Autodesk Fusion 360 part; units mm, degrees
sketch "Sketch1" plane through (0, 0, 0) normal (0, 1, 0) x (1, 0, 0)
  circle A0 centre (0, 0) radius 71.65
  circle A1 centre (0, 0) radius 83.65
  circle A2 centre (0, 0) radius 86.15 construction
  line L0 (0, 0) -> (10, 0) construction
  line L1 (-106.5, 0) -> (126.5, 0) construction
  line L2 (-84.5, -69.5) -> (104.5, -69.5) construction
  line L3 (104.5, -69.5) -> (104.5, 69.5) construction
  line L4 (104.5, 69.5) -> (-84.5, 69.5) construction
  line L5 (-84.5, 69.5) -> (-84.5, -69.5) construction
  line L6 (-84.5, -69.5) -> (104.5, 69.5) construction
  line L7 (104.5, -69.5) -> (-84.5, 69.5) construction
  line L8 (93.5, -59) -> (-73.5, -59) construction
  line L9 (-73.5, -59) -> (-73.5, 59) construction
  line L10 (-73.5, 59) -> (93.5, 59) construction
  line L11 (93.5, 59) -> (93.5, -59) construction
  line L12 (93.5, -59) -> (-73.5, 59) construction
  line L13 (-73.5, -59) -> (93.5, 59) construction
  line L14 (0, 86.15) -> (0, -86.15) construction
  circle A3 centre (0, 0) radius 77.65 construction
  line L15 (0, 0) -> (54.9068, -54.9068) construction
  line L16 (0, 0) -> (77.65, 0) construction
  point P0 (10, 0)
  point P1 (10, 0)
  dimension "d1" = 143.3
  dimension "d2" = 167.3
  dimension "d3" = 172.3
  dimension "d5" = 10
  dimension "d6" = 233
  dimension "d7" = 189
  dimension "d8" = 139
  dimension "d9" = 167
  dimension "d10" = 118
  dimension "d22" = 155.3
  dimension "d23" = 45
sketch "Sketch2" plane through (0, 0, 0) normal (0, 1, 0) x (1, 0, 0)
  spline S0 degree 5 poles (-84.5, 69.5) (-81.1215, 70.7869) (-74.3286, 73.2455) (-64.0315, 76.5883) (-50.083, 80.3433) (-32.2585, 83.7904) (-14.0132, 85.8889) (4.6825, 86.5435) (23.8364, 85.73) (43.4214, 83.5343) (63.4013, 80.0731) (79.6732, 76.3808) (92.0287, 73.1261) (100.3319, 70.7441) (104.5, 69.5) knots 0 0 0 0 0 0 0.1 0.2 0.3 0.4 0.5 0.6 0.7 0.8 0.9 1 1 1 1 1 1
  line L0 (104.5, 69.5) -> (-84.5, 69.5)
  spline S1 degree 5 poles (-84.5, -69.5) (-81.1215, -70.7869) (-74.3286, -73.2455) (-64.0315, -76.5883) (-50.083, -80.3433) (-32.2585, -83.7904) (-14.0132, -85.8889) (4.6825, -86.5435) (23.8364, -85.73) (43.4214, -83.5343) (63.4013, -80.0731) (79.6732, -76.3808) (92.0287, -73.1261) (100.3319, -70.7441) (104.5, -69.5) knots 0 0 0 0 0 0 0.1 0.2 0.3 0.4 0.5 0.6 0.7 0.8 0.9 1 1 1 1 1 1
  line L1 (104.5, -69.5) -> (104.5, 69.5)
  spline S2 degree 5 poles (-84.5, 69.5) (-86.1686, 66.72) (-89.3602, 61.16) (-93.7104, 52.82) (-98.6219, 41.7) (-103.1794, 27.8) (-106.0136, 13.9) (-106.9839, 0) (-106.0136, -13.9) (-103.1794, -27.8) (-98.6219, -41.7) (-93.7104, -52.82) (-89.3602, -61.16) (-86.1686, -66.72) (-84.5, -69.5) knots 0 0 0 0 0 0 0.1 0.2 0.3 0.4 0.5 0.6 0.7 0.8 0.9 1 1 1 1 1 1
  spline S3 degree 5 poles (104.5, 69.5) (106.1686, 66.72) (109.3602, 61.16) (113.7104, 52.82) (118.6219, 41.7) (123.1794, 27.8) (126.0136, 13.9) (126.9839, 0) (126.0136, -13.9) (123.1794, -27.8) (118.6219, -41.7) (113.7104, -52.82) (109.3602, -61.16) (106.1686, -66.72) (104.5, -69.5) knots 0 0 0 0 0 0 0.1 0.2 0.3 0.4 0.5 0.6 0.7 0.8 0.9 1 1 1 1 1 1
  point P0 (0, 86.15)
  point P1 (-84.5, 69.5)
  point P2 (0, 86.15)
  point P3 (104.5, 69.5)
  point P4 (0, -86.15)
  point P5 (-84.5, -69.5)
  point P6 (0, -86.15)
  point P7 (104.5, -69.5)
  point P8 (-106.5, 0)
  point P9 (-106.5, 0)
  point P10 (126.5, 0)
  point P11 (126.5, 0)
sketch "Sketch3" plane through (0, 0, 0) normal (0, 1, 0) x (1, 0, 0)
  line L0 (-77.5372, 58.4854) -> (-72.637, 55.023)
  arc A0 (-72.637, 55.023) -> (-69.4632, 59.5149) centre (-71.0501, 57.2689) ccw
  line L1 (-69.4632, 59.5149) -> (-74.3634, 62.9773)
  arc A1 (-74.3634, 62.9773) -> (-77.5372, 58.4854) centre (-75.9503, 60.7313) ccw
  line L2 (-75.9503, 60.7313) -> (-71.0501, 57.2689) construction
  line L3 (93.5, -59) -> (-73.5, 59)
  line L4 (-73.5, -59) -> (93.5, 59)
  line L5 (94.3632, 62.9771) -> (89.463, 59.5147)
  arc A2 (89.463, 59.5147) -> (92.6368, 55.0229) centre (91.0499, 57.2688) ccw
  line L6 (92.6368, 55.0229) -> (97.537, 58.4853)
  arc A3 (97.537, 58.4853) -> (94.3632, 62.9771) centre (95.9501, 60.7312) ccw
  line L7 (95.9501, 60.7312) -> (91.0499, 57.2688) construction
  line L8 (97.537, -58.4853) -> (92.6368, -55.0229)
  arc A4 (92.6368, -55.0229) -> (89.463, -59.5147) centre (91.0499, -57.2688) ccw
  line L9 (89.463, -59.5147) -> (94.3632, -62.9771)
  arc A5 (94.3632, -62.9771) -> (97.537, -58.4853) centre (95.9501, -60.7312) ccw
  line L10 (95.9501, -60.7312) -> (91.0499, -57.2688) construction
  line L11 (-74.3632, -62.9771) -> (-69.463, -59.5147)
  arc A6 (-69.463, -59.5147) -> (-72.6368, -55.0229) centre (-71.0499, -57.2688) ccw
  line L12 (-72.6368, -55.0229) -> (-77.537, -58.4853)
  arc A7 (-77.537, -58.4853) -> (-74.3632, -62.9771) centre (-75.9501, -60.7312) ccw
  line L13 (-75.9501, -60.7312) -> (-71.0499, -57.2688) construction
  line L14 (-80.541, 57.6998) -> (-72.374, 51.9291)
  arc A8 (-72.374, 51.9291) -> (-66.459, 60.3002) centre (-69.4165, 56.1147) ccw
  line L15 (-66.459, 60.3002) -> (-74.626, 66.0709)
  arc A9 (-74.626, 66.0709) -> (-80.541, 57.6998) centre (-77.5835, 61.8853) ccw
  line L16 (-77.5835, 61.8853) -> (-69.4165, 56.1147) construction
  line L17 (94.571, 66.032) -> (86.404, 60.2613)
  arc A10 (86.404, 60.2613) -> (92.3189, 51.8902) centre (89.3615, 56.0758) ccw
  line L18 (92.3189, 51.8902) -> (100.4859, 57.6609)
  arc A11 (100.4859, 57.6609) -> (94.571, 66.032) centre (97.5284, 61.8464) ccw
  line L19 (97.5284, 61.8464) -> (89.3615, 56.0758) construction
  line L20 (100.541, -57.6998) -> (92.374, -51.9291)
  arc A12 (92.374, -51.9291) -> (86.459, -60.3002) centre (89.4165, -56.1147) ccw
  line L21 (86.459, -60.3002) -> (94.626, -66.0709)
  arc A13 (94.626, -66.0709) -> (100.541, -57.6998) centre (97.5835, -61.8853) ccw
  line L22 (97.5835, -61.8853) -> (89.4165, -56.1147) construction
  line L23 (-74.626, -66.0709) -> (-66.459, -60.3002)
  arc A14 (-66.459, -60.3002) -> (-72.374, -51.9291) centre (-69.4165, -56.1147) ccw
  line L24 (-72.374, -51.9291) -> (-80.541, -57.6998)
  arc A15 (-80.541, -57.6998) -> (-74.626, -66.0709) centre (-77.5835, -61.8853) ccw
  line L25 (-77.5835, -61.8853) -> (-69.4165, -56.1147) construction
  point P0 (-73.5002, 59.0001)
  point P1 (93.5, 59)
  point P2 (93.5, -59)
  point P3 (-73.5, -59)
  point P4 (-73.5, 59)
  point P5 (93.4449, 58.9611)
  point P6 (93.5, -59)
  point P7 (-73.5, -59)
  dimension "d12" = 3
  dimension "d13" = 5.5
  dimension "d16" = 5.5
  dimension "d17" = 3
  dimension "d18" = 3
  dimension "d19" = 5.5
  dimension "d20" = 3
  dimension "d21" = 5.5
  dimension "d30" = 10.25
  dimension "d31" = 10.25
  dimension "d32" = 10.25
  dimension "d33" = 10.25
sketch "Sketch4" plane through (0, 0, 0) normal (0, 1, 0) x (1, 0, 0)
  circle A0 centre (54.9068, -54.9068) radius 2.625
  circle A1 centre (54.9068, -54.9068) radius 6
  circle A2 centre (54.9068, 54.9068) radius 2.625
  circle A3 centre (54.9068, 54.9068) radius 6
  circle A4 centre (-54.9068, 54.9068) radius 2.625
  circle A5 centre (-54.9068, 54.9068) radius 6
  circle A6 centre (-54.9068, -54.9068) radius 2.625
  circle A7 centre (-54.9068, -54.9068) radius 6
  point P0 (54.9068, -54.9068)
  dimension "d24" = 5.25
  dimension "d25" = 12
  dimension "d27" = 360
extrude "Extrude1" add sketch "Sketch2" against normal blind 6
extrude "Extrude4" cut sketch "Sketch3" sketch "Sketch4" sketch "Sketch1" along normal up to surface contours L0 A0 L1 A1 | L5 A2 L6 A3 | L8 A4 L9 A5 | L11 A6 L12 A7 of sketch 2 contours A0 | A2 | A4 | A6 of sketch 3 contours A0 end surface through (0, -6, 0) normal (0, -1, 0) offset 0
fillet "Fillet2" radius 65 4 edges at (104.5, -3, 69.5) (104.5, -3, -69.5) (-84.5, -3, 69.5) (-84.5, -3, -69.5)
The model under review builds one solid part; all positions refer to its coordinate system, in mm. Round coordinates to 2 decimals unless told otherwise and drop trailing zeros.
Item 1: Mouldability with a two-part tool opening along X and no side actions: class faces 1 (the face through (88.77, -2.96, -55.73)), 2 (the face through (-55.476, -2.958, -52.344)), 3 (the face through (60, 0, -40)) as released by +X, released by -X, zero draft, split by the parting line, or undercut.
Determined:
face 1: undercut
face 2: undercut
face 3: zero draft
Item 2: For line 1 (Z direction, x = 90, y = -4.25); line 2 (X direction, y = -2.25, z = -55); line 3 (Z direction, x = 0, y = -3.9), list the stretches that pass through material, from the lowest coordinate up.
Determined:
line 1: z = -71.42 to -59.89, -54.73 to 54.73, 59.89 to 71.42
line 2: x = -90.41 to -72.6, -69.5 to -57.53, -52.28 to -45.92, 45.92 to 52.28, 57.53 to 89.5, 92.6 to 109.67
line 3: z = -86.15 to -71.65, 71.65 to 86.15
Item 3: Clearance check with flat-ended pins moving along their axes: pin 1 Ø7 at (x, z) = (-54.91, 54.91) entering from -Y; pin 2 Ø1 at (y, z) = (-4, 52) entering from +X; pin 3 Ø2 at (x, y) = (97.5, -1) entering from -Z; pin 4 Ø2 at (x, y) = (17.5, -3) entering from +Z. State where each tip first meets the part, or that it passes through.
Determined:
pin 1: stops at y = -6
pin 2: stops at x = 112.29
pin 3: stops at z = -67.38
pin 4: stops at z = 85.86
Item 4: Take a section at A-A (y = -4.25). Give the number of separate pieces and of enclosed holes in the cut face, then the cut area to 3 significant figures.
Determined:
separate pieces: 1
enclosed holes: 9
area: 17,500 mm2
